from build123d import *

# Parameters (mm, degrees)
BOSS_EXTRUDE1_DEPTH = 4
CUT_EXTRUDE2_DEPTH  = 4
SKETCH5_W           = 4
SKETCH5_H           = 30
BOSS_EXTRUDE2_DEPTH = 30


with BuildPart() as part:
    # Sketch1 → Boss-Extrude1 (new body)
    with BuildSketch(Plane.XY):
        Polygon((0, 0), (-38.149545772, 0), (-38.149545772, -4), (-58.149545772, -4), (-58.149545772, 0), (-98.149545772, 0), (-46.188021545, 30), (-11.547005384, 30), (-20.207259423, 45.000000002), (-11.547005385, 50.000000002), (0, 30), align=None)
    extrude(amount=BOSS_EXTRUDE1_DEPTH)

    # Sketch3 → Cut-Extrude2 (cut)
    with BuildSketch(Plane.XY.offset(4)):
        with BuildLine():
            Line((-6.593479065, 35.551516575), (-10.950440862, 43.025442617))
            ThreePointArc((-10.950440862, 43.025442617), (-14.369311445, 43.926177837), (-15.270046665, 40.507307254))
            Line((-15.270046665, 40.507307254), (-10.913084868, 33.033381213))
            ThreePointArc((-10.913084868, 33.033381213), (-7.494214285, 32.132645993), (-6.593479065, 35.551516575))
        make_face()
    extrude(amount=-CUT_EXTRUDE2_DEPTH, mode=Mode.SUBTRACT)

    # Sketch5 → Boss-Extrude2 (add)
    with BuildSketch(Plane(origin=(0, 0, 0), x_dir=(0, 0, -1), z_dir=(1, 0, 0))):
        with Locations((-2, 15)):
            Rectangle(SKETCH5_W, SKETCH5_H)
    extrude(amount=BOSS_EXTRUDE2_DEPTH)


solid = part.part
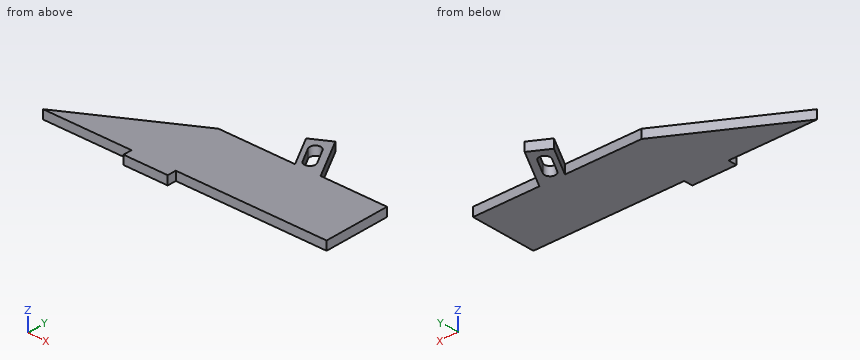
Part model, mm, in its own coordinate system. Coordinates: 2 decimals unless noted, no trailing zeros. Loops run counter-clockwise (first coordinate to the right, second up) from the corner with the lowest first, then second, coordinate; pieces in that order, holes last. Notation, with made-up numbers: (45, 88.25) -> (70, 88.25) arc R32 cw to (70, 122.25) -> close; hole circle Ø11 at (34, 75). An arc over 180 degrees is marked (long way). Use a Markdown table: item, result. Add a question column.
Item 1: Band-saw the part on B-B on x = 20. Write the cut outline in (y, z).
Item 2: Band-saw the part on A-A on z = 2.8. Write the cut outline in (x, y).
Item 3: Band-saw the part on C-C on y = 21. Write the cut outline in (x, z).
Item 4: Probe probe 1 along Y at (x, z) = (-41, 3.55); probe 2 along Y at (x, z) = (-11, 1); probe 3 along X at (y, z) = (43, 3.7). List the from-to ranges inside material, lowest first.
Item 5: Flat gauge pins, fed straight in: P1, Ø1, axis at x = -83.5, z = 2, coming from the +Y side; P2, Ø1.2, axis at x = 16, z = 1, coming from the +Y side; P3, Ø2, axis at y = -2, z = 3, coming from the -X side; P4, Ø10, axis at x = -44.5, y = 37, coming from the -Z side. Where does each tip first touch, or does it go through?
Geometry says:
| question | item | result |
|---|---|---|
| 1 | outline | (0, 0) -> (30, 0) -> (30, 4) -> (0, 4) -> close |
| 2 | outline | (-98.15, 0) -> (-58.15, 0) -> (-58.15, -4) -> (-38.15, -4) -> (-38.15, 0) -> (30, 0) -> (30, 30) -> (0, 30) -> (-11.55, 50) -> (-20.21, 45) -> (-11.55, 30) -> (-46.19, 30) -> close; hole (-15.27, 40.51) -> (-10.91, 33.03) arc R2.5 ccw to (-6.59, 35.55) -> (-10.95, 43.03) arc R2.5 ccw to start |
| 3 | outline | (-61.78, 0) -> (30, 0) -> (30, 4) -> (-61.78, 4) -> close |
| 4 | probe 1 | -4 to 30 |
| 4 | probe 2 | 0 to 33.18, 43.11 to 49.05 |
| 4 | probe 3 | -19.05 to -15.28, -10.94 to -7.51 |
| 5 | P1 | y = 8.75 |
| 5 | P2 | y = 30 |
| 5 | P3 | x = -58.15 |
| 5 | P4 | through |
